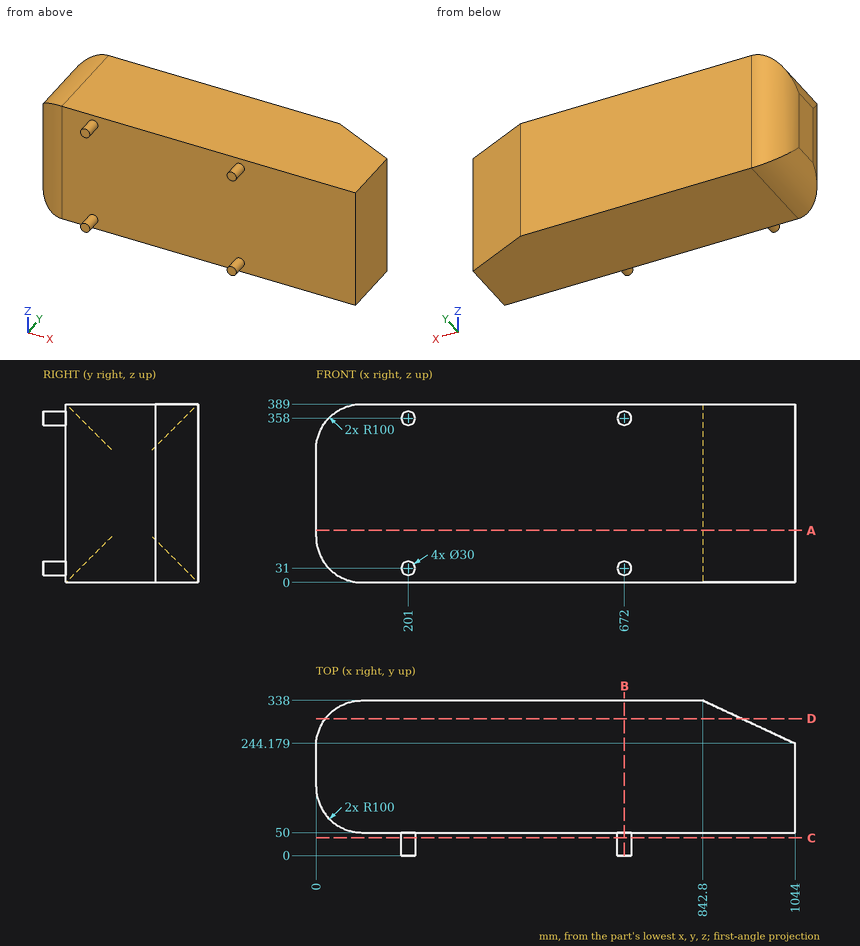
Geometry: see drawing. Coordinates: mm, zero at the bounding-box minimum. Coordinates: 2 decimals unless noted, no trailing zeros. Order: outer loops, then holes, each group sorted by start corner. A loop starts at its lowest first (then second) coordinate and runs counter-clockwise, first axis right, second up. Notation, with made-up numbers: (-36.75, 13) -> (-19.75, 13) arc R5 ccw to (-19.75, 19) -> close; hole circle Ø2 at (6, 27). An arc over 180 degrees is marked (long way). Write each question's results on one line, items separated by ' | '. Start each with the question number.
1) Material intervals for line 1 along Y through (x, z) = (293, 195); line 2 along X through (y, z) = (136.5, 343.5) (1 decimal); line 3 along Y through (x, z) = (875.5, 139), sorted ascending.
2) First-contact query: pin 1 (3 mm diameter, centred on x = 905, z = 182.5, fed in from -Y); pin 2 (4 mm diameter, centred on y = 169, z = 248.5, fed in from -X); pin 3 (1.5 mm diameter, centred on y = 89, z = 186.5, fed in from -X); pin 4 (4 mm diameter, centred on y = 249, z = 341.5, fed in from +X). Flat tips, straight axial feed; report the tip coordinate or a pass-through.
3) Cut plane D-D, the plane y = 298.5. Output: boundary loops of the cut face in (x, z), and give its area (3 significant figures).
4) Cut plane A-A, the plane z = 113.5. Output: boundary loops of the cut face in (x, y).
5) Cut plane B-B, the plane x = 672. Output: boundary loops of the cut face in (y, z), and give its area (3 significant figures).
6) Cut plane C-C, the plane y = 38.5. Output: boundary loops of the cut face in (x, z).
Checks:
1) line 1: 50 to 338 | line 2: 16.2 to 1044 | line 3: 50 to 322.75
2) pin 1: y = 50 | pin 2: x = 0 | pin 3: x = 20.19 | pin 4: x = 1037.95
3) outline: (20.38, 39.5) arc R100 ccw to (100, 0) -> (927.51, 0) -> (927.51, 389) -> (100, 389) arc R100 ccw to (20.38, 349.5) -> close | area: 351,000 mm^2
4) outline: (0, 150) arc R100 ccw to (100, 50) -> (1044, 50) -> (1044, 244.18) -> (842.8, 338) -> (100, 338) arc R100 ccw to (0, 238) -> close
5) outline: (0, 16) -> (50, 16) -> (50, 0) -> (338, 0) -> (338, 389) -> (50, 389) -> (50, 373) -> (0, 373) -> (0, 343) -> (50, 343) -> (50, 46) -> (0, 46) -> close | area: 115,000 mm^2
6) outline: circle Ø30 at (201, 31); circle Ø30 at (201, 358); circle Ø30 at (672, 31); circle Ø30 at (672, 358)
